The listing builds one solid part. Answer for the finished solid, in the listing's coordinates (mm). A direction names the side the tool comes from. Round coordinates to 2 decimals unless told otherwise and drop trailing zeros. Loops run counter-clockwise (first coordinate to the right, second up) from the corner with the lowest first, then second, coordinate; pieces in that order, holes last. Notation, with made-up numbers: (79, 23) -> (136, 23) arc R28 ccw to (136, 59) -> close; hole circle Ø1 at (5.5, 67.5). An arc over 180 degrees is marked (long way). Write each question's results on one line, items separated by ' | '. Start each with the question number.
from build123d import *

# Parameters (mm, degrees)
PAD_DEPTH = 10
FILLET_R  = 1


with BuildPart() as part:
    # Sketch → Pad (new body)
    with BuildSketch(Plane.XY):
        with BuildLine():
            Line((-1.4, 4), (-1.4, -1))
            Line((-1.4, -1), (-2.4, -1))
            ThreePointArc((-2.4, -1), (-6.642641, -2.757359), (-8.4, -7))
            Line((-8.4, -7), (-8.4, -26))
            ThreePointArc((-8.4, -26), (-7.298979, -29.464102), (-4.4, -31.656854))
            Line((-4.4, -31.656854), (-4.4, -33))
            Line((-6.4, -35), (-4.4, -33))
            Line((-6.4, -35), (-6.4, -36))
            Line((-6.4, -36), (-4.4, -38))
            Line((-4.4, -38), (-2.4, -38))
            Line((-2.4, -29), (-2.4, -38))
            ThreePointArc((-5.4, -26), (-4.52132, -28.12132), (-2.4, -29))
            Line((-5.4, -7), (-5.4, -26))
            ThreePointArc((-2.4, -4), (-4.52132, -4.87868), (-5.4, -7))
            Line((1.4, -4), (-2.4, -4))
            Line((1.4, -4), (1.4, 4))
            Line((1.4, 4), (1.9, 7))
            Line((1.9, 7), (-1.9, 7))
            Line((-1.9, 7), (-1.4, 4))
        make_face()
    extrude(amount=PAD_DEPTH)

    # Fillet
    fillet_edges = [part.edges().sort_by_distance(p)[0] for p in [
        (1.4, -4, 5),
        (-2.4, -29, 5),
    ]]
    fillet(fillet_edges, radius=FILLET_R)


solid = part.part
Item 1: Straight lines are drawn through the part: L1, parallel to Y at x = -0.5, z = 2.5; L2, parallel to X at y = -14, z = 3.25; L3, parallel to Y at x = -4, z = 5.75. For each, find the intervals that lie inside material, in ascending order. Write a range as [from, to].
Item 2: The part is cut by section A-A, the plane z = 2.25. Give the vertices of the cut face in (x, y), plus the area to 3 significant figures.
Item 3: Determine the mould class of faces 5 (the cylindrical face through (1.099, -3.715, 5.07)), 6 (the flat face through (-5.4, -34, 4.9)), 7 (the flat face through (1.4, 0, 5)) for opening direction Y: +Y half, -Y half, draft (parallel to the pull), parting line (faces both ways), or undercut.
Item 4: The part is cut by section B-B, the plane x = -4. Give the vertices of the cut face in (y, z), plus the area to 3 significant figures.
Item 5: The part is cut by section C-C, the plane y = 2. Give the vertices of the cut face in (x, z), plus the area to 3 significant figures.
Item 6: Each of these flat-tipped pins is pushed along its axis until it touches: pin 1 Ø6 at (x, z) = (-6.5, 5.5) entering from +Y; pin 2 Ø5.5 at (y, z) = (1.5, 4) entering from +X; pin 3 Ø2.5 at (y, z) = (2.5, 5.5) entering from -X. Where does it stop, or does it pass through?
Item 7: For faces 1 (the flat face through (-4.4, -32, 5)), 2 (the flat face through (-1, -4, 5)), 3 (the cylindrical face through (-4.8, -27.8, 4.9)), 4 (the flat face through (-6.4, -35.5, 4.9)), determine the directions among +Z, -Z, +X, -X, +Y, -Y from which every point of the face is accessible in a straight line to the end or side of a thin tool.
Item 8: The part is cut by section D-D, the plane x = -0.25. Give the vertices of the cut face in (y, z), plus the area to 3 significant figures.
Report:
1) L1: y = [-4, 7] | L2: x = [-8.4, -5.4] | L3: y = [-38, -28.54], [-4.46, -1.22]
2) outline: (-8.4, -26) arc R6 ccw to (-4.4, -31.66) -> (-4.4, -33) -> (-6.4, -35) -> (-6.4, -36) -> (-4.4, -38) -> (-2.4, -38) -> (-2.4, -29.87) arc R1 ccw to (-3.15, -28.9) arc R3 cw to (-5.4, -26) -> (-5.4, -7) arc R3 cw to (-2.4, -4) -> (0.4, -4) arc R1 ccw to (1.4, -3) -> (1.4, 4) -> (1.9, 7) -> (-1.9, 7) -> (-1.4, 4) -> (-1.4, -1) -> (-2.4, -1) arc R6 ccw to (-8.4, -7) -> close | area: 153 mm2
3) face 5: -Y half | face 6: undercut | face 7: draft
4) outline: (-38, 0) -> (-28.54, 0) -> (-28.54, 10) -> (-38, 10) -> close; (-4.46, 0) -> (-1.22, 0) -> (-1.22, 10) -> (-4.46, 10) -> close | area: 127 mm2
5) outline: (-1.4, 0) -> (1.4, 0) -> (1.4, 10) -> (-1.4, 10) -> close | area: 28.0 mm2
6) pin 1: stops at y = -1.1 | pin 2: stops at x = 1.44 | pin 3: stops at x = -1.4
7) face 1: +Z, -Z, -X | face 2: +Z, -Z, +X, -Y | face 3: +Z, -Z, +X | face 4: +Z, -Z, -X, -Y
8) outline: (-4, 0) -> (7, 0) -> (7, 10) -> (-4, 10) -> close | area: 110 mm2
